Can you work these out from the model? Positions are in its coordinate system, mm. Face numbers are marked on the shaded views. A direction names the side the tool comes from. Give positions to 0.01 mm unless a question says otherwise; leave off trailing zeros. Write each loop counter-clockwise with the first axis right and the second up, starting at its lowest first coordinate (ties: lowest second). Pieces come first, ordered by that corner, then holes. Notation, with made-up numbers: M -5,61 L 13,61 A23 cw 13,93 Z; hole C 25,14.25 d4. An arc over 180 degrees is marked long. Use CSV: the item, a comma, the result in double quotes. Start each with the question number.
from build123d import *

# Parameters (mm, degrees)
SALIENTE_EXTRUIR1_DEPTH = 6
SALIENTE_EXTRUIR2_DEPTH = 32
CORTAR_EXTRUIR1_REACH   = 39.705
CROQUIS3_R              = 9.5
CORTAR_EXTRUIR2_DEPTH   = 31


with BuildPart() as part:
    # Croquis1 → Saliente-Extruir1 (new body)
    with BuildSketch(Plane.XY):
        with BuildLine():
            Line((-22, 17), (-22, -15))
            Line((-22, -15), (-14, -15))
            Line((-14, -15), (-14, 0))
            ThreePointArc((-14, 0), (0, 14), (14, 0))
            Line((14, 0), (14, -15))
            Line((14, -15), (22, -15))
            Line((22, -15), (22, 17))
            Line((22, 17), (-22, 17))
        make_face()
    extrude(amount=SALIENTE_EXTRUIR1_DEPTH)

    # Croquis2 → Saliente-Extruir2 (add)
    with BuildSketch(Plane.XZ.offset(15)):
        Polygon((22, 6), (22, 9.32233047), (4.32233047, 27), (2.201010127, 24.878679656), (17.757359313, 9.32233047), (17.757359313, 6), align=None)
    extrude(amount=-SALIENTE_EXTRUIR2_DEPTH)

    # Croquis3 → Cortar-Extruir1 (cut, up to next)
    with BuildSketch(Plane(origin=(15.661165235, 0, 15.661165235), x_dir=(0.707106781, 0, -0.707106781), z_dir=(0.707106781, 0, 0.707106781)), mode=Mode.PRIVATE) as cortar_extruir1_sk1:
        with Locations((-3.535533906, 0)):
            Circle(CROQUIS3_R)
    cortar_extruir1_tool1 = extrude(cortar_extruir1_sk1.sketch, amount=-CORTAR_EXTRUIR1_REACH, mode=Mode.PRIVATE) & part.part
    add(cortar_extruir1_tool1.solids().sort_by_distance((13.161165, 0, 18.161165))[0], mode=Mode.SUBTRACT)

    # Croquis5 → Cortar-Extruir2 (cut)
    with BuildSketch(Plane(origin=(0, 17, 0), x_dir=(1, 0, 0), z_dir=(0, 1, 0))):
        Polygon((4.499107166, -25.232233047), (20.232233047, -9.499107166), (19.701902961, -8.96877708), (3.96877708, -24.701902961), align=None)
    extrude(amount=-CORTAR_EXTRUIR2_DEPTH, mode=Mode.SUBTRACT)


solid = part.part
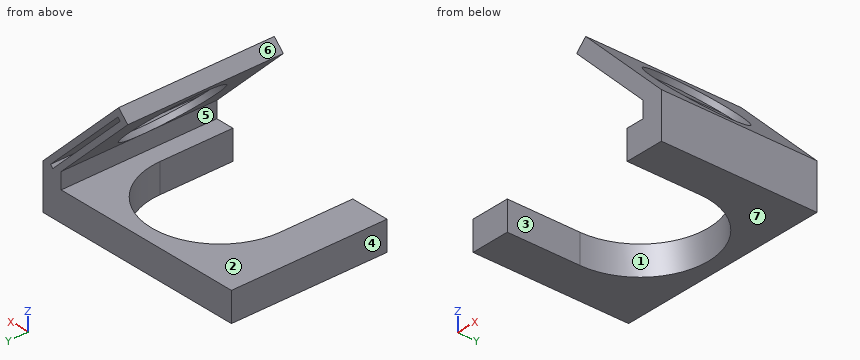
(1) Please list where these lines run through material, in increasing order: L1, parallel to X at y = -4, z = 3; L2, parallel to X at y = -8, z = 7.25; L3, parallel to Z at x = 13, y = -11. Write a range as [from, to].
(2) I want a section at D-D (x = 0). Write out the boundary of the cut face in (y, z).
(3) Which directions (+Z, -Z, +X, -X, +Y, -Y) give clear straight access to the entire face, cutting with the end or side of a thin tool? Please do the marked faces 1, 2, 3 and 4.
(4) I want a section at B-B (y = 5.5). Write out the boundary of the cut face in (x, z), and give its area (3 significant figures).
(5) Thinking about a two-plate mould opening in Z: for the marked faces 5, 6 and 7, which applies, released by +Z, released by -Z, zero draft, split by the parting line, or undercut?
(6) I want a section at C-C (x = 14.5). State how many separate pieces and enclosed holes the cut face has, and give its area (3 significant figures).
(7) Will these pins go through, and if not, where does the flat tip stop? pin 1 Ø1 at (y, z) = (3.5, 8.5) entering from -X; pin 2 Ø2 at (y, z) = (1.5, 14.5) entering from +X; pin 3 Ø3 at (y, z) = (6, 11) entering from -X; pin 4 Ø12 at (y, z) = (5, 18.5) entering from +X.
(8) I want a section at A-A (y = 12). Write out the boundary of the cut face in (x, z).
Geometry results:
1,L1,"x = [-22, -14], [14, 22]"
1,L2,"x = [17.76, 22]"
1,L3,"z = [14.08, 15.67], [16.73, 18.32]"
2,outline,"M 14,0 L 17,0 L 17,6 L 14,6 Z"
3,face 1,"-Z, -Y"
3,face 2,"-X, +Y, -Y"
3,face 3,"+Z, -Z, -Y"
3,face 4,"+Z, -Z, -X, +Y, -Y"
4,outline,"M -22,0 L -12.87,0 L -12.87,6 L -22,6 Z; M 2.2,24.88 L 5.56,21.52 L 6.36,22.31 L 3.97,24.7 L 4.5,25.23 L 6.89,22.84 L 7.68,23.64 L 4.32,27 Z; M 12.87,0 L 22,0 L 22,9.32 L 18.64,12.68 L 17.84,11.89 L 20.23,9.5 L 19.7,8.97 L 17.31,11.36 L 16.52,10.56 L 17.76,9.32 L 17.76,6 L 12.87,6 Z"
4,area,"143 mm2"
5,face 5,"undercut"
5,face 6,"released by +Z"
5,face 7,"released by -Z"
6,separate pieces,"4"
6,enclosed holes,"0"
6,area,"239 mm2"
7,pin 1,"stops at x = 17.76"
7,pin 2,"passes through"
7,pin 3,"stops at x = 15.34"
7,pin 4,"stops at x = 18.82"
8,outline,"M -22,0 L -7.21,0 L -7.21,6 L -22,6 Z; M 2.2,24.88 L 17.76,9.32 L 17.76,6 L 7.21,6 L 7.21,0 L 22,0 L 22,9.32 L 4.32,27 Z; hole M 3.97,24.7 L 19.7,8.97 L 20.23,9.5 L 4.5,25.23 Z"
